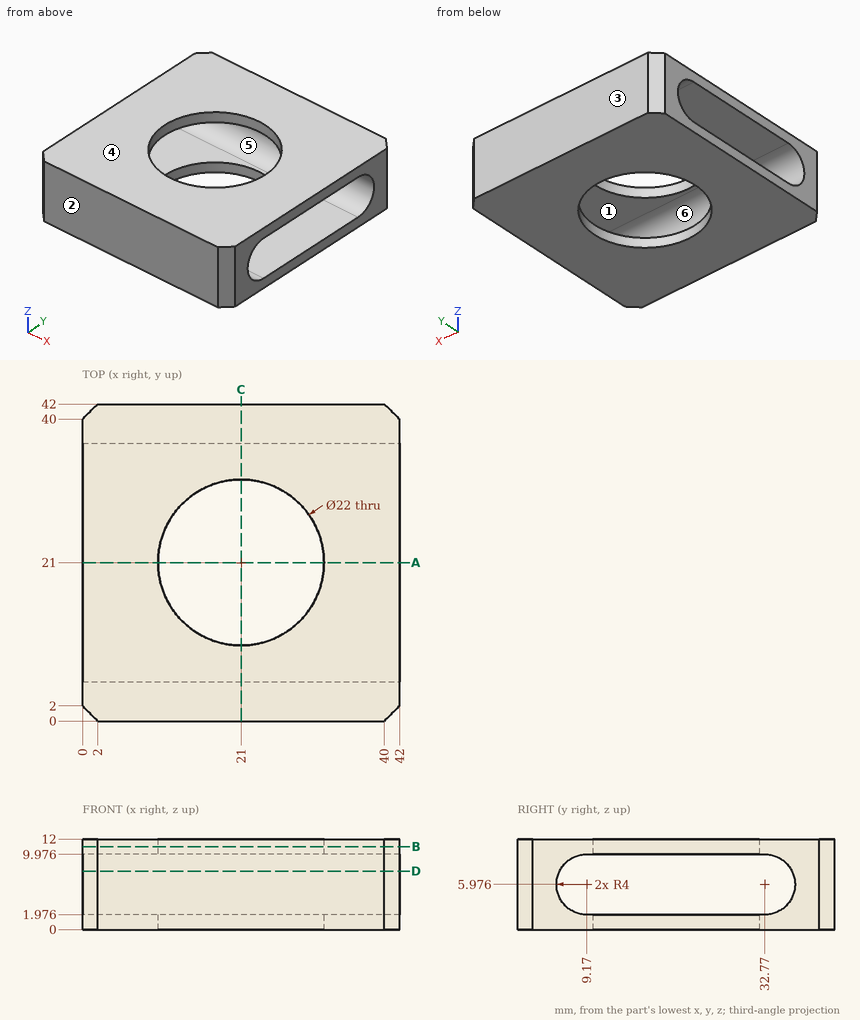
Design review of the part shown in the three views and the two pictorial views. Dimensions are in mm from the part's minimum x, y and z. A direction names the side the tool comes from. Coordinates: 2 decimals unless noted, no trailing zeros. Write each loop counter-clockwise with the first axis right and the second up, starting at its lowest first coordinate (ties: lowest second). Pieces come first, ordered by that corner, then holes. Notation, with made-up numbers: (-11.5, -38) - (17.5, -38) arc R26 cw to (17.5, -9) - close; hole circle Ø1 at (15, 29.5). An arc over 180 degrees is marked (long way). Write item = value, one per line.
(1) Consider section B-B, the plane z = 11. Give the boundary of the cut face in (x, y).
Result sheet:
outline = (0, 2) - (2, 0) - (40, 0) - (42, 2) - (42, 40) - (40, 42) - (2, 42) - (0, 40) - close; hole circle Ø22 at (21, 21)
(2) For line 1 (X direction, y = 21, z = 0.4); line 2 (Z direction, x = 40, y = 12.5), list the stretches that pass through material, from the lowest coordinate up. Write a range as [from, to].
Result sheet:
line_1 = [0, 10], [32, 42]
line_2 = [0, 1.98], [9.98, 12]
(3) Consider section D-D, the plane z = 7.75. Give the boundary of the cut face in (x, y) (1 decimal).
Result sheet:
outline = (0, 2) - (2, 0) - (40, 0) - (42, 2) - (42, 5.6) - (0, 5.6) - close; (0, 36.4) - (42, 36.4) - (42, 40) - (40, 42) - (2, 42) - (0, 40) - close
(4) Machinability: for the marked faces 1 and 2, which of the approach directions +Z, -Z, +X, -X, +Y, -Y give a long, thin tool a straight path to every point of the face, cutting with its end or side? Answer none if there is none.
Result sheet:
face_1 = +X, -X
face_2 = +Z, -Z, +X, -X, -Y
(5) For P1, Ø13, axis at x = 21, y = 21, coming from the +Z side, flat-tipped, find the tip position at first contact; note if it passes through.
Result sheet:
P1 = through
(6) Mouldability with a two-part tool opening along Z and no side actions: class the marked faces 3, 4, 5 and 6 as pulls with the +Z half, pulls with the -Z half, needs draft (parallel to the pull), parting line crosses it, or undercut.
Result sheet:
face_3 = needs draft
face_4 = pulls with the +Z half
face_5 = undercut
face_6 = undercut
(7) Consider section A-A, the plane y = 21. Give the boundary of the cut face in (x, z).
Result sheet:
outline = (0, 0) - (10, 0) - (10, 1.98) - (0, 1.98) - close; (0, 9.98) - (10, 9.98) - (10, 12) - (0, 12) - close; (32, 0) - (42, 0) - (42, 1.98) - (32, 1.98) - close; (32, 9.98) - (42, 9.98) - (42, 12) - (32, 12) - close
(8) Consider section C-C, the plane x = 21. Give the boundary of the cut face in (y, z), then the cut area to 3 significant figures.
Result sheet:
outline = (0, 0) - (10, 0) - (10, 1.98) - (9.17, 1.98) arc R4 cw to (9.17, 9.98) - (10, 9.98) - (10, 12) - (0, 12) - close; (32, 0) - (42, 0) - (42, 12) - (32, 12) - (32, 9.98) - (32.77, 9.98) arc R4 cw to (32.77, 1.98) - (32, 1.98) - close
area = 177 mm^2
